CAD build for the part. Positions are in the model's coordinates, mm. Face numbers are marked on the shaded views. A direction names the side the tool comes from. Coordinates: 2 decimals unless noted, no trailing zeros. Order: outer loops, then holes, each group sorted by start corner. A loop starts at its lowest first (then second) coordinate and runs counter-clockwise, first axis right, second up. Notation, with made-up numbers: (-32.5, 48) - (1.5, 48) arc R6 ccw to (1.5, 52) - close; hole circle Ø1 at (11, 36). An arc over 180 degrees is marked (long way). Write each question's results on one line, items separated by ' | '. Start each with the question number.
Q1. Pull direction X, two halves, no side cores. Call the marked faces 6, 7 and 8: released by +X, released by -X, zero draft, split by the parting line, or undercut.
Q2. Band-saw the part on D-D, the plane x = 12. Write the cut outline in (y, z), then the cut area to 3 significant figures.
Q3. Which spindle directions (+Z, -Z, +X, -X, +Y, -Y) get a long thin tool onto all of the face, cutting with end or side? Do the marked faces 1, 2, 3, 4 and 5. Say none if no direction does.
Q4. Band-saw the part on C-C, the plane y = 2.7. Write the cut outline in (x, z).
Q5. Wall check: probe 1 along Z at (x, y) = (18.5, 1.35); probe 2 along Z at (x, y) = (3, 0.2); probe 3 along Z at (x, y) = (7, 2.3). Give the ranges that are in metal, low to high.
Q6. Band-saw the part on B-B, the plane x = 5.7. Write the cut outline in (y, z), then the cut area to 3 significant figures.
Q7. Pin check, flat tips, straight feed: P1, Ø1.5, axis at x = 20, y = 1, coming from the -Z side; P2, Ø1.5, axis at y = 2, z = -6, coming from the -X side; P3, Ø1.5, axis at x = 1.5, y = 1, coming from the +Z side. Stop position of each tip, or through.
Q8. Band-saw the part on A-A, the plane z = -5. Write the cut outline in (x, y).
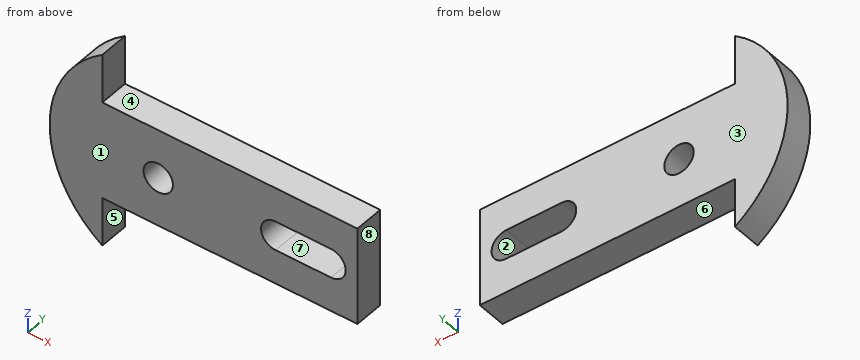
Autodesk Inventor part; units mm, degrees
ref_plane "YZ Plane" through (0, 0, 0) normal (1, 0, 0) x (0, 1, 0)
ref_plane "XZ Plane" through (0, 0, 0) normal (0, 1, 0) x (-1, 0, 0)
ref_plane "XY Plane" through (0, 0, 0) normal (0, 0, 1) x (1, 0, 0)
sketch "Sketch1" plane through (0, 0, 0) normal (0, 1, 0) x (-1, 0, 0)
  line L0 (0, 0) -> (-26, 0)
  line L1 (-26, 0) -> (-26, -10)
  line L2 (-26, -10) -> (0, -10)
  line L3 (0, -10) -> (0, 0)
  line L4 (0, 0) -> (0, 5)
  line L5 (0, -10) -> (0, -15)
  circle A0 centre (-5.7, -5) radius 1.5
  arc A1 (-23.3, -3.5) -> (-23.3, -6.5) centre (-23.3, -5) ccw
  line L6 (-23.3, -3.5) -> (-17.6724, -3.5)
  line L7 (-17.6724, -3.5) -> (-17.6724, -6.5)
  line L8 (-17.6724, -6.5) -> (-23.3, -6.5)
  arc A2 (-17.6724, -6.5) -> (-17.6724, -3.5) centre (-17.6724, -5) ccw
  arc A3 (0, -15) -> (0, 5) centre (-6.6332, -5) ccw
  dimension "d0" = 26
  dimension "d1" = 10
  dimension "d5" = 3
  dimension "d7" = 3
  dimension "d8" = 3
  dimension "d9" = 12
extrude "Extrusion1" add sketch "Sketch1" along normal blind 3
properties part number "FPV_Motor_Holder"
Results below:
1) face 6: zero draft | face 7: undercut | face 8: released by +X
2) outline: (0, -10) - (3, -10) - (3, 0) - (0, 0) - close | area: 30.0 mm²
3) face 1: +Z, -Z, +X, -X, -Y | face 2: +Y, -Y | face 3: +Z, -Z, +X, -X, +Y | face 4: +Z, +X, +Y, -Y | face 5: -Z, +X, +Y, -Y
4) outline: (0, -15) - (0, -10) - (26, -10) - (26, 0) - (0, 0) - (0, 5) arc R12 ccw to start; hole circle Ø3 at (5.7, -5); hole (17.67, -6.5) - (23.3, -6.5) arc R1.5 ccw to (23.3, -3.5) - (17.67, -3.5) arc R1.5 ccw to start
5) probe 1: z = -10 to -6.5, -3.5 to 0 | probe 2: z = -10 to 0 | probe 3: z = -10 to -5.75, -4.25 to 0
6) outline: (0, -10) - (3, -10) - (3, -6.5) - (0, -6.5) - close; (0, -3.5) - (3, -3.5) - (3, 0) - (0, 0) - close | area: 21.0 mm²
7) P1: stops at z = -10 | P2: stops at x = -5.36 | P3: stops at z = 0
8) outline: (-5.37, 0) - (4.2, 0) - (4.2, 3) - (-5.37, 3) - close; (7.2, 0) - (16.17, 0) - (16.17, 3) - (7.2, 3) - close; (24.8, 0) - (26, 0) - (26, 3) - (24.8, 3) - close
